Read the model definition and answer for the solid it produces. Units are mm, in the model's axes. A direction names the side the tool comes from. Coordinates: 2 decimals unless noted, no trailing zeros. Write each loop counter-clockwise with the first axis right and the second up, starting at its lowest first coordinate (ties: lowest second). Pieces come first, ordered by that corner, then holes.
(1) Given pin 1 (11 mm diameter, centred on x = -14.5, z = 23.5, fed in from -Y); pin 2 (3 mm diameter, centred on x = -14.5, z = 24.5, fed in from +Y); pin 3 (9 mm diameter, centred on x = 31.5, z = -0.5, fed in from -Y); pin 4 (1.5 mm diameter, centred on y = 55, z = -14.5, fed in from +X), each flat-ended and moving along its own axis, determine where each tip first touches the part or whether it passes through.
(2) Which of the six approach directions +Z, -Z, +X, -X, +Y, -Y give full straight-line access (tool end or side, diameter ignored) to faces 1 (the flat face through (-10, 70, -10)), 2 (the cylindrical face through (11.923, -16.902, 3.755)), 3 (the flat face through (15, -9.5, -26)), 4 (the flat face through (-15, -0.5, 26)), 5 (the flat face through (0.43, -36.82, 7.99))?
(3) The mould has two halves that part along Y. Classify faces 6 (the flat face through (11.2, 0, 6.1)), 7 (the cylindrical face through (11.923, 83.944, 3.755)), 8 (the flat face through (-6.1, -10, -11.2)): +Y half, -Y half, draft (parallel to the pull), parting line (faces both ways), or undercut.
(4) Find the intervals of material crossed by probe 1 along Y at (x, z) = (11, -14); probe 2 along Y at (x, z) = (9.5, -4.5); probe 3 along Y at (x, z) = (-24.5, 14.5), in increasing order.
(5) Section A-A on y = -38.5 is taken. Write down the section's boundary in (x, z), then the cut area to 3 significant figures.
(6) Section B-B on y = 32 is taken. Write down the section's boundary in (x, z), then the cut area to 3 significant figures.
from build123d import *

# Parameters (mm, degrees)
F0_R      = 26
F1_DEPTH  = 10
F4_DEPTH  = 4.5
F5_R      = 1
F6_COUNT  = 12
F7_R      = 12.5
F8_DEPTH  = 98
F9_DEPTH  = 14
F11_DEPTH = 26
F13_R     = 26
F14_DEPTH = 5
F15_SIZE  = 2


with BuildPart() as f1:
    # F0 (on Front) → F1 (new body)
    with BuildSketch(Plane.XZ):
        Circle(F0_R)
    extrude(amount=F1_DEPTH)

    # F3 (on mid) → F4 (join, symmetric)
    with BuildSketch(Plane.XZ.offset(5)):
        with BuildLine():
            Line((-35.9444015112, -2), (-25.6904651573, -4))
            Line((-25.6904651573, -4), (-25.6904651573, 4))
            Line((-25.6904651573, 4), (-35.9444015112, 2))
            ThreePointArc((-35.9444015112, 2), (-36, 0), (-35.9444015112, -2))
        make_face()
    extrude(amount=F4_DEPTH, both=True)

    # F5
    f5_edges = [f1.edges().sort_by_distance(p)[0] for p in [
        (-35.944402, -5, -2),
        (-35.944402, -5, 2),
    ]]
    fillet(f5_edges, radius=F5_R)


with BuildPart() as f6_1:
    # F6: instance of F1
    add(f1.part.rotate(Axis((0, 0, 0), (0, -1, 0)), 1 * 360 / F6_COUNT))


with BuildPart() as f6_2:
    # F6: instance of F1
    add(f1.part.rotate(Axis((0, 0, 0), (0, -1, 0)), 2 * 360 / F6_COUNT))


with BuildPart() as f6_3:
    # F6: instance of F1
    add(f1.part.rotate(Axis((0, 0, 0), (0, -1, 0)), 3 * 360 / F6_COUNT))


with BuildPart() as f6_4:
    # F6: instance of F1
    add(f1.part.rotate(Axis((0, 0, 0), (0, -1, 0)), 4 * 360 / F6_COUNT))


with BuildPart() as f6_5:
    # F6: instance of F1
    add(f1.part.rotate(Axis((0, 0, 0), (0, -1, 0)), 5 * 360 / F6_COUNT))


with BuildPart() as f6_6:
    # F6: instance of F1
    add(f1.part.rotate(Axis((0, 0, 0), (0, -1, 0)), 6 * 360 / F6_COUNT))


with BuildPart() as f6_7:
    # F6: instance of F1
    add(f1.part.rotate(Axis((0, 0, 0), (0, -1, 0)), 7 * 360 / F6_COUNT))


with BuildPart() as f6_8:
    # F6: instance of F1
    add(f1.part.rotate(Axis((0, 0, 0), (0, -1, 0)), 8 * 360 / F6_COUNT))


with BuildPart() as f6_9:
    # F6: instance of F1
    add(f1.part.rotate(Axis((0, 0, 0), (0, -1, 0)), 9 * 360 / F6_COUNT))


with BuildPart() as f6_10:
    # F6: instance of F1
    add(f1.part.rotate(Axis((0, 0, 0), (0, -1, 0)), 10 * 360 / F6_COUNT))


with BuildPart() as f6_11:
    # F6: instance of F1
    add(f1.part.rotate(Axis((0, 0, 0), (0, -1, 0)), 11 * 360 / F6_COUNT))


with BuildPart() as f8:
    # F7 (on face) → F8 (new body)
    with BuildSketch(Plane.XZ.offset(10)):
        Circle(F7_R)
    extrude(amount=-F8_DEPTH)


with BuildPart() as f9:
    # F9 (new): a face of the model
    f9_faces = [f8.part.faces().sort_by_distance(p)[0] for p in [
        (0, -10, 0),
    ]]
    extrude(f9_faces, amount=F9_DEPTH)

    # F10 (on face) → F11 (join)
    with BuildSketch(Plane.XZ.offset(24)):
        Polygon((8.7402150444, 1.5656130559), (4.2253893698, 7.8095190592), (-3.4712406825, 8.1726979258), (-8.5539557005, 2.3816685616), (-7.1953676071, -5.2028058067), (-0.4185209468, -8.8694612846), (6.6734805227, -5.8572315112), align=None)
    extrude(amount=F11_DEPTH)


with BuildPart() as f1_1:
    add(f1.part)

    add(f6_1.part)  # F14 merges F6_1

    add(f6_2.part)  # F14 merges F6_2

    add(f6_3.part)  # F14 merges F6_3

    add(f6_4.part)  # F14 merges F6_4

    add(f6_5.part)  # F14 merges F6_5

    add(f6_6.part)  # F14 merges F6_6

    add(f6_7.part)  # F14 merges F6_7

    add(f6_8.part)  # F14 merges F6_8

    add(f6_9.part)  # F14 merges F6_9

    add(f6_10.part)  # F14 merges F6_10

    add(f6_11.part)  # F14 merges F6_11

    add(f8.part)  # F14 merges F8

    add(f9.part)  # F14 merges F9
    # F13 (on offset) → F14 (join, symmetric)
    with BuildSketch(Plane(origin=(0, 75, 0), x_dir=(-1, 0, 0), z_dir=(0, 1, 0))):
        Circle(F13_R)
    extrude(amount=F14_DEPTH, both=True)

    # F15
    f15_edges = [f1_1.edges().sort_by_distance(p)[0] for p in [
        (26, 80, 0),
        (26, 70, 0),
    ]]
    chamfer(f15_edges, length=F15_SIZE)


solid = f1_1.part
Response:
1. pin 1: stops at y = -10
1. pin 2: stops at y = -0.5
1. pin 3: stops at y = -9.5
1. pin 4: passes through
2. face 1: none
2. face 2: -Y
2. face 3: -Z, +X, -Y
2. face 4: +Z, -X, +Y
2. face 5: +Z, +X, -Y
3. face 6: undercut
3. face 7: draft
3. face 8: -Y half
4. probe 1: y = -10 to 0, 70 to 80
4. probe 2: y = -24 to 88
4. probe 3: y = -9.5 to -0.5
5. outline: (-8.55, 2.38) - (-7.2, -5.2) - (-0.42, -8.87) - (6.67, -5.86) - (8.74, 1.57) - (4.23, 7.81) - (-3.47, 8.17) - close
5. area: 216 mm2
6. outline: circle Ø25 at (0, 0)
6. area: 491 mm2
